Work out the finished part from the listing and answer in its coordinate system (mm). A direction names the side the tool comes from. Round coordinates to 2 decimals unless told otherwise and drop trailing zeros. Loops run counter-clockwise (first coordinate to the right, second up) from the corner with the lowest first, then second, coordinate; pieces in that order, holes last. Notation, with made-up numbers: (89.25, -28) - (117.25, -28) arc R12 cw to (117.25, -19) - close; hole circle Ø10 at (41.5, -3.5). An arc over 180 degrees is marked (long way). Return JSON: item names as keys, results as strings.
from build123d import *

# Parameters (mm, degrees)
EXTRUDE1_DEPTH = 2
EXTRUDE2_DEPTH = 0.1
EXTRUDE3_DEPTH = 0.1


with BuildPart() as part:
    # Sketch1 → Extrude1 (new body)
    with BuildSketch(Plane.XY):
        with BuildLine():
            Line((-50, 5), (50, 5))
            ThreePointArc((50, 5), (55, 0), (50, -5))
            Line((50, -5), (-50, -5))
            ThreePointArc((-50, -5), (-55, 0), (-50, 5))
        make_face()
    extrude(amount=EXTRUDE1_DEPTH)

    # Sketch2 → Extrude2 (add)
    with BuildSketch(Plane.XY.offset(2)):
        with BuildLine():
            Line((-50, 5), (50, 5))
            ThreePointArc((50, 5), (55, 0), (50, -5))
            Line((50, -5), (-50, -5))
            ThreePointArc((-50, -5), (-55, 0), (-50, 5))
        make_face()
        with BuildLine():
            Line((-50, 4), (50, 4))
            ThreePointArc((50, 4), (54, 0), (50, -4))
            Line((50, -4), (-50, -4))
            ThreePointArc((-50, -4), (-54, 0), (-50, 4))
        make_face(mode=Mode.SUBTRACT)
    extrude(amount=EXTRUDE2_DEPTH)

    # Sketch3 → Extrude3 (add)
    with BuildSketch(Plane.XY.offset(2)):
        with BuildLine():
            Line((-49.999999498, 2), (-32.499999623, 2))
            ThreePointArc((-32.499999623, 2), (-30.499999623, 0), (-32.499999623, -2))
            Line((-32.499999623, -2), (-49.999999498, -2))
            ThreePointArc((-49.999999498, -2), (-51.999999498, 0), (-49.999999498, 2))
        make_face()
        with BuildLine():
            Line((-50, 1.8), (-32.499999623, 1.8))
            ThreePointArc((-32.499999623, 1.8), (-30.699999623, 0), (-32.499999623, -1.8))
            Line((-32.499999623, -1.8), (-50, -1.8))
            ThreePointArc((-50, -1.8), (-51.8, 0), (-50, 1.8))
        make_face(mode=Mode.SUBTRACT)
        with BuildLine():
            Line((-22.499999623, 2), (-4.999999749, 2))
            ThreePointArc((-4.999999749, 2), (-2.999999749, 0), (-4.999999749, -2))
            Line((-4.999999749, -2), (-22.499999623, -2))
            ThreePointArc((-22.499999623, -2), (-24.499999623, 0), (-22.499999623, 2))
        make_face()
        with BuildLine():
            Line((-22.499999623, 1.8), (-4.999999749, 1.8))
            ThreePointArc((-4.999999749, 1.8), (-3.199999749, 0), (-4.999999749, -1.8))
            Line((-4.999999749, -1.8), (-22.499999623, -1.8))
            ThreePointArc((-22.499999623, -1.8), (-24.299999623, 0), (-22.499999623, 1.8))
        make_face(mode=Mode.SUBTRACT)
        with BuildLine():
            Line((5.000000251, 2), (22.500000126, 2))
            ThreePointArc((22.500000126, 2), (24.500000126, 0), (22.500000126, -2))
            Line((22.500000126, -2), (5.000000251, -2))
            ThreePointArc((5.000000251, -2), (3.000000251, 0), (5.000000251, 2))
        make_face()
        with BuildLine():
            Line((5.000000251, 1.8), (22.500000126, 1.8))
            ThreePointArc((22.500000126, 1.8), (24.300000126, 0), (22.500000126, -1.8))
            Line((22.500000126, -1.8), (5.000000251, -1.8))
            ThreePointArc((5.000000251, -1.8), (3.200000251, 0), (5.000000251, 1.8))
        make_face(mode=Mode.SUBTRACT)
        with BuildLine():
            Line((32.500000126, 2), (50, 2))
            ThreePointArc((50, 2), (52, 0), (50, -2))
            Line((50, -2), (32.500000126, -2))
            ThreePointArc((32.500000126, -2), (30.500000126, 0), (32.500000126, 2))
        make_face()
        with BuildLine():
            Line((32.500000126, 1.8), (50, 1.8))
            ThreePointArc((50, 1.8), (51.8, 0), (50, -1.8))
            Line((50, -1.8), (32.500000126, -1.8))
            ThreePointArc((32.500000126, -1.8), (30.700000126, 0), (32.500000126, 1.8))
        make_face(mode=Mode.SUBTRACT)
    extrude(amount=EXTRUDE3_DEPTH)


solid = part.part
1) Section C-C (y = -3) is taken. Give the vertices of the cut face in (x, z).
Verdict:
{"outline": "(-54, 0) - (54, 0) - (54, 2.1) - (52.65, 2.1) - (52.65, 2) - (-52.65, 2) - (-52.65, 2.1) - (-54, 2.1) - close"}
2) Determine the mould class of faces 1 (the flat face through (1, 0, 2)), 2 (the cylindrical face through (55, 0, 1)), 3 (the flat face through (1, -5, 1)) for opening direction X: pulls with the +X half, pulls with the -X half, needs draft (parallel to the pull), parting line crosses it, or undercut.
Verdict:
{"face 1": "undercut", "face 2": "pulls with the +X half", "face 3": "needs draft"}
3) Section B-B (z = 1.4) is taken. Give the vertices of the cut face in (x, y), and give its area (3 significant figures).
Verdict:
{"outline": "(-50, -5) - (50, -5) arc R5 ccw to (50, 5) - (-50, 5) arc R5 ccw to start", "area": "1,080 mm2"}
4) A flat-ended cylindrical pin translates along its axis: pin 1 (3 mm diameter, centred on x = -42.5, y = 0, fed in from +Z). Find the tip coordinate at first contact, or state that the pin passes through.
Verdict:
{"pin 1": "stops at z = 2"}
5) Find the intervals of material crossed by L1, parallel to Z at x = 10.5, y = 2.25; L2, parallel to X at y = -0.5, z = 0.75; L3, parallel to X at y = -4.5, z = 1, in increasing order.
Verdict:
{"L1": "z = 0 to 2", "L2": "x = -54.97 to 54.97", "L3": "x = -52.18 to 52.18"}
6) A tool of negligible diameter and unlimited length cuts with its end or side. For faces 4 (the flat face through (1, 0, 0)), 5 (the flat face through (14, 0, 2)), from which of +Z, -Z, +X, -X, +Y, -Y can it reach the whole face along a straight path? Write none if from no direction.
Verdict:
{"face 4": "-Z, +X, -X, +Y, -Y", "face 5": "+Z"}
7) Section A-A (x = -10) is taken. Give the vertices of the cut face in (y, z).
Verdict:
{"outline": "(-5, 0) - (5, 0) - (5, 2.1) - (4, 2.1) - (4, 2) - (2, 2) - (2, 2.1) - (1.8, 2.1) - (1.8, 2) - (-1.8, 2) - (-1.8, 2.1) - (-2, 2.1) - (-2, 2) - (-4, 2) - (-4, 2.1) - (-5, 2.1) - close"}
